```python
from build123d import *

# Parameters (mm, degrees)
SKETCH5_R          = 2
CUT_EXTRUDE4_DEPTH = 18
SKETCH6_R          = 2
CUT_EXTRUDE5_DEPTH = 18


with BuildPart() as part:
    # Sketch1 → Revolve1 (revolve)
    with BuildSketch(Plane.XY, mode=Mode.PRIVATE) as revolve1_sk:
        Polygon((4, 0), (15, 0), (15, 7.5), (22, 7.5), (22, 9.25), (20.69, 9.25), (20.69, 26.25), (22, 26.25), (22, 28), (4, 28), align=None)
    revolve(revolve1_sk.sketch.rotate(Axis((0, 0, 0), (0, 1, 0)), 90), axis=Axis((0, 0, 0), (0, 1, 0)))

    # Sketch5 → Cut-Extrude4 (cut)
    with BuildSketch(Plane.XY):
        with Locations(Location((0, 3.526654559, 0), (0, 0, 270.000000001))):
            Circle(SKETCH5_R)
    extrude(amount=-CUT_EXTRUDE4_DEPTH, mode=Mode.SUBTRACT)

    # Sketch6 → Cut-Extrude5 (cut)
    with BuildSketch(Plane(origin=(0, 0, 0), x_dir=(0, 0, -1), z_dir=(1, 0, 0))):
        with Locations((0, 3.75)):
            Circle(SKETCH6_R)
    extrude(amount=-CUT_EXTRUDE5_DEPTH, mode=Mode.SUBTRACT)


solid = part.part
```
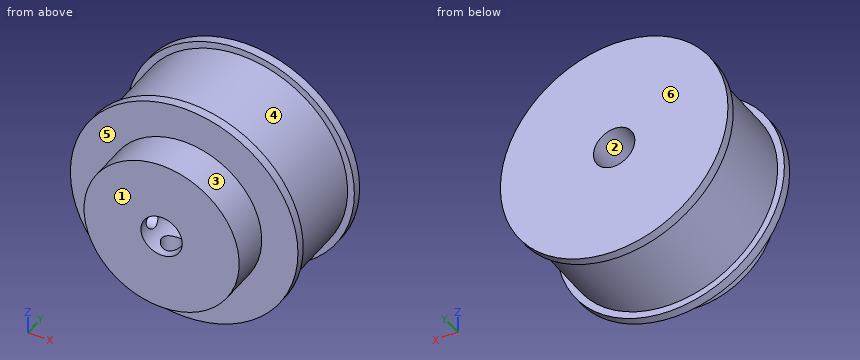
Part model, mm, in its own coordinate system. Face numbers are marked on the shaded views. A direction names the side the tool comes from. Round coordinates to 2 decimals unless told otherwise and drop trailing zeros. Write each loop counter-clockwise with the first axis right and the second up, starting at its lowest first coordinate (ties: lowest second). Pieces come first, ordered by that corner, then holes. Notation, with made-up numbers: (4.25, 28) -> (59.25, 28) arc R20 ccw to (59.25, 32) -> close; hole circle Ø8 at (28.25, 79). An arc over 180 degrees is marked (long way). Return JSON: item names as keys, results as strings. Group by question number.
Q1. Probe L1, parallel to X at y = 20.75, z = 0; L2, parallel to Y at x = -9.25, z = 0; L3, parallel to X at y = 7, z = 0. List the from-to ranges inside material, lowest first. Write a range as [from, to].
Q2. Mould opens along Z. For the marked faces 1, 2 and 3 say: pulls with the +Z half, pulls with the -Z half, needs draft (parallel to the pull), parting line crosses it, or undercut.
Q3. Saw through at D-D on x = -13.5. Write the cut outline in (y, z).
Q4. Which spindle directions (+Z, -Z, +X, -X, +Y, -Y) get a long thin tool onto all of the face, cutting with end or side? Do the marked faces 4, 5 and 6. Say none if no direction does.
Q5. Saw through at C-C on y = 3. Write the cut outline in (x, z).
Q6. Saw through at B-B on z = 0. Write the cut outline in (x, y), plus the area to 3 significant figures.
Q7. Saw through at A-A on x = 0. Write the cut outline in (y, z), plus the area to 3 significant figures.
Q8. Pin check, flat tips, straight feed: pin 1 (12 mm diameter, centred on y = 24, z = -8, fed in from +X); pin 2 (3.5 mm diameter, centred on x = 0, y = 3.53, fed in from -Z); pin 3 (4 mm diameter, centred on y = 12.5, z = -11.5, fed in from +X). Stop position of each tip, or through.
Answer:
{
 "1": {"L1": "[-20.69, -4], [4, 20.69]", "L2": "[0, 1.75], [5.75, 28]", "L3": "[-15, -4], [4, 15]"},
 "2": {"face 1": "needs draft", "face 2": "undercut", "face 3": "parting line crosses it"},
 "3": {"outline": "(0, -6.54) -> (7.5, -6.54) -> (7.5, -17.37) -> (9.25, -17.37) -> (9.25, -15.68) -> (26.25, -15.68) -> (26.25, -17.37) -> (28, -17.37) -> (28, 17.37) -> (26.25, 17.37) -> (26.25, 15.68) -> (9.25, 15.68) -> (9.25, 17.37) -> (7.5, 17.37) -> (7.5, 6.54) -> (0, 6.54) -> close; hole circle Ø4 at (3.75, 0)"},
 "4": {"face 4": "none", "face 5": "-Y", "face 6": "+Z, -Z, +X, -X, +Y"},
 "5": {"outline": "(-14.88, -1.85) arc R15 ccw to (-1.93, -14.88) -> (-1.93, -3.5) arc R4 cw to (-3.54, -1.85) -> close; (-14.88, 1.85) -> (-3.54, 1.85) arc R4 cw (long way) to (1.93, -3.5) -> (1.93, -14.88) arc R15 ccw (long way) to start"},
 "6": {"outline": "(-22, 7.5) -> (-15, 7.5) -> (-15, 5.75) -> (-4, 5.75) -> (-4, 28) -> (-22, 28) -> (-22, 26.25) -> (-20.69, 26.25) -> (-20.69, 9.25) -> (-22, 9.25) -> close; (-15, 0) -> (-4, 0) -> (-4, 1.75) -> (-15, 1.75) -> close; (4, 0) -> (15, 0) -> (15, 7.5) -> (22, 7.5) -> (22, 9.25) -> (20.69, 9.25) -> (20.69, 26.25) -> (22, 26.25) -> (22, 28) -> (4, 28) -> close", "area": "814 mm2"},
 "7": {"outline": "(0, -15) -> (1.53, -15) -> (1.53, -4) -> (0, -4) -> close; (0, 4) -> (28, 4) -> (28, 22) -> (26.25, 22) -> (26.25, 20.69) -> (9.25, 20.69) -> (9.25, 22) -> (7.5, 22) -> (7.5, 15) -> (0, 15) -> close; (5.53, -15) -> (7.5, -15) -> (7.5, -22) -> (9.25, -22) -> (9.25, -20.69) -> (26.25, -20.69) -> (26.25, -22) -> (28, -22) -> (28, -4) -> (5.53, -4) -> close", "area": "814 mm2"},
 "8": {"pin 1": "x = 21.86", "pin 2": "z = 3.6", "pin 3": "x = 18.38"}
}
